Design review of the part built by this model. Coordinates are the model's own, in mm. A direction names the side the tool comes from. Coordinates: 2 decimals unless noted, no trailing zeros. Order: outer loops, then holes, each group sorted by start corner. A loop starts at its lowest first (then second) coordinate and runs counter-clockwise, first axis right, second up. Notation, with made-up numbers: M 6.5,24.25 L 44.5,24.25 A23 cw 44.5,36.25 Z; hole C 59,-13 d5. An arc over 180 degrees is marked long. Answer in a Markdown table with one row per item.
from build123d import *

# Parameters (mm, degrees)
SKETCH_1_W          = 30
SKETCH_1_H          = 20
EXTRUDE_1_DEPTH     = 3
SKETCH_2_R          = 1.6
CUT_EXTRUDE_1_DEPTH = 19.275666882
SKETCH_3_W          = 15
SKETCH_3_H          = 30
SKETCH_3_R          = 1.45
EXTRUDE_2_DEPTH     = 3
SKETCH_4_W          = 30
SKETCH_4_H          = 6
CUT_EXTRUDE_2_DEPTH = 34.674916481
SKETCH_5_R          = 1.45
SKETCH_5_R_2        = 2.6
EXTRUDE_3_DEPTH     = 3
CUT_EXTRUDE_3_DEPTH = 43.532340636
FILLET_1_R          = 3


with BuildPart() as part:
    # 草图1 → 凸台-拉伸1 (new body)
    with BuildSketch(Plane(origin=(0, 0, 0), x_dir=(1, 0, 0), z_dir=(0, 1, 0))):
        Rectangle(SKETCH_1_W, SKETCH_1_H)
    extrude(amount=EXTRUDE_1_DEPTH)

    # 草图2 → 切除-拉伸1 (cut, through all)
    with BuildSketch(Plane(origin=(0, 3, 0), x_dir=(1, 0, 0), z_dir=(0, 1, 0))):
        with Locations(Location((-5, 7.5, 0), (0, 0, 270))):
            Circle(SKETCH_2_R)
        with Locations(Location((5, 7.5, 0), (0, 0, 270))):
            Circle(SKETCH_2_R)
        with Locations(Location((5, -7.5, 0), (0, 0, 270))):
            Circle(SKETCH_2_R)
        with Locations(Location((-5, -7.5, 0), (0, 0, 270))):
            Circle(SKETCH_2_R)
    extrude(amount=-CUT_EXTRUDE_1_DEPTH, mode=Mode.SUBTRACT)

    # 草图3 → 凸台-拉伸2 (add)
    # profile 1 of 2: a face of its own
    with BuildSketch(Plane(origin=(0, 3, 0), x_dir=(1, 0, 0), z_dir=(0, 1, 0))):
        with Locations((22.5, 0)):
            Rectangle(SKETCH_3_W, SKETCH_3_H)
        with Locations(Location((22.5, -10, 0), (0, 0, 90))):
            Circle(SKETCH_3_R, mode=Mode.SUBTRACT)
        with Locations(Location((22.5, 10, 0), (0, 0, 90))):
            Circle(SKETCH_3_R, mode=Mode.SUBTRACT)
    # profile 2 of 2: a face of its own
    with BuildSketch(Plane(origin=(0, 3, 0), x_dir=(1, 0, 0), z_dir=(0, 1, 0))):
        with Locations((-22.5, 0)):
            Rectangle(SKETCH_3_W, SKETCH_3_H)
        with Locations(Location((-22.5, 10, 0), (0, 0, 270))):
            Circle(SKETCH_3_R, mode=Mode.SUBTRACT)
        with Locations(Location((-22.5, -10, 0), (0, 0, 270))):
            Circle(SKETCH_3_R, mode=Mode.SUBTRACT)
    extrude(amount=-EXTRUDE_2_DEPTH)

    # 草图4 → 切除-拉伸2 (cut, through all)
    with BuildSketch(Plane.XZ):
        with Locations((0, 7)):
            Rectangle(SKETCH_4_W, SKETCH_4_H)
        with Locations((0, -7)):
            Rectangle(SKETCH_4_W, SKETCH_4_H)
    extrude(amount=-CUT_EXTRUDE_2_DEPTH, mode=Mode.SUBTRACT)

    # 草图5 → 凸台-拉伸3 (add)
    with BuildSketch(Plane(origin=(0, 3, 0), x_dir=(1, 0, 0), z_dir=(0, 1, 0))):
        Polygon((30, -15), (15, -15), (-15, -15), (-30, -15), (-30, -30), (30, -30), align=None)
        with Locations(Location((-10, -22.5, 0), (0, 0, 270))):
            Circle(SKETCH_5_R, mode=Mode.SUBTRACT)
        with Locations(Location((0, -22.5, 0), (0, 0, 270))):
            Circle(SKETCH_5_R_2, mode=Mode.SUBTRACT)
        with Locations(Location((10, -22.5, 0), (0, 0, 270))):
            Circle(SKETCH_5_R, mode=Mode.SUBTRACT)
    extrude(amount=-EXTRUDE_3_DEPTH)

    # 草图6 → 切除-拉伸3 (cut, through all)
    with BuildSketch(Plane(origin=(0, 3, 0), x_dir=(1, 0, 0), z_dir=(0, 1, 0))):
        Polygon((-30, -15), (-15, -30), (-30, -30), align=None)
        Polygon((30, -30), (30, -15), (15, -30), align=None)
    extrude(amount=-CUT_EXTRUDE_3_DEPTH, mode=Mode.SUBTRACT)

    # 圆角1
    fillet_1_edges = [part.edges().sort_by_distance(p)[0] for p in [
        (-30, 1.5, 15),
        (-15, 1.5, 30),
        (15, 1.5, 30),
        (30, 1.5, 15),
        (15, 1.5, 15),
        (15, 1.5, -15),
        (30, 1.5, -15),
        (-15, 1.5, -15),
        (-15, 1.5, 15),
        (-30, 1.5, -15),
        (-15, 1.5, 4),
        (15, 1.5, 4),
        (-15, 1.5, -4),
        (15, 1.5, -4),
    ]]
    fillet(fillet_1_edges, radius=FILLET_1_R)


solid = part.part
(1) Add section A-A, the plane x = -22.5. Give the boundary of the cut face in (y, z), and give its area (3 significant figures).
Return value:
| item | result |
|---|---|
| outline | M 0,-15 L 3,-15 L 3,-11.45 L 0,-11.45 Z; M 0,-8.55 L 3,-8.55 L 3,8.55 L 0,8.55 Z; M 0,11.45 L 3,11.45 L 3,22.5 L 0,22.5 Z |
| area | 95.1 mm2 |
(2) Insertion check: pin 1 Ø12 at (x, z) = (-3, 5) entering from +Y; pin 2 Ø1.5 at (x, y) = (-5.5, 1) entering from -Z. Each pin has a flat end and moves straight along its axis. Give the tip position at first contact, or say it passes through.
Return value:
| item | result |
|---|---|
| pin 1 | stops at y = 3 |
| pin 2 | stops at z = -4 |
(3) Add section B-B, the plane z = 10. Give the boundary of the cut face in (x, y), and give its area (3 significant figures).
Return value:
| item | result |
|---|---|
| outline | M -30,0 L -23.95,0 L -23.95,3 L -30,3 Z; M -21.05,0 L -15,0 L -15,3 L -21.05,3 Z; M 15,0 L 21.05,0 L 21.05,3 L 15,3 Z; M 23.95,0 L 30,0 L 30,3 L 23.95,3 Z |
| area | 72.6 mm2 |
(4) For faces 5 (the cylindrical face through (-29.765, 1.479, 14.921)), 6 (the cylindrical face through (14.1, 1.48, 14.14)), 7 (the flat face through (-15, 2, -9)), list the 3-axis set-ups (+Z, -Z, +X, -X, +Y, -Y) from which the entire face can be reached by the end or side of a thin tool; tool diameter is ignored.
Return value:
| item | result |
|---|---|
| face 5 | +Z, -X, +Y, -Y |
| face 6 | +Y, -Y |
| face 7 | -Z, +Y, -Y |
(5) Draft analysis for pull direction X (two halves, no side actions). For faces 1 (the flat face through (0, 2, 30)), 2 (the cylindrical face through (0.78, 1.52, 24.98)), 3 (the cylindrical face through (29.765, 1.479, 14.921)), 4 (the flat face through (0, 1, 4)), state which applies: pulls with the +X half, pulls with the -X half, needs draft (parallel to the pull), parting line crosses it, or undercut.
Return value:
| item | result |
|---|---|
| face 1 | needs draft |
| face 2 | undercut |
| face 3 | pulls with the +X half |
| face 4 | undercut |
(6) Add section C-C, the plane z = -6. Give the boundary of the cut face in (x, y).
Return value:
| item | result |
|---|---|
| outline | M -30,0 L -14.83,0 L -14.83,3 L -30,3 Z; M 14.83,0 L 30,0 L 30,3 L 14.83,3 Z |
(7) For line 1 along X through (y, z) = (1.95, 10); line 2 along Z through (x, y) = (12, 2.6); line 3 along Z through (x, y) = (22.5, 1.25), list the stretches that pass through material, from the lowest coordinate up. Write a range as from..to.
Return value:
| item | result |
|---|---|
| line 1 | x = -30..-23.95, -21.05..-15, 15..21.05, 23.95..30 |
| line 2 | z = -4..4, 15..30 |
| line 3 | z = -15..-11.45, -8.55..8.55, 11.45..22.5 |
